Geometry check sheet. Reference: the model listing, model coordinates, mm. A direction names the side the tool comes from. Coordinates: 2 decimals unless noted, no trailing zeros. Order: outer loops, then holes, each group sorted by start corner. A loop starts at its lowest first (then second) coordinate and runs counter-clockwise, first axis right, second up. Notation, with made-up numbers: (88, -31) -> (111, -31) arc R6 ccw to (111, -26) -> close; hole circle Ø10 at (-9, -18). An arc over 180 degrees is marked (long way). Answer as CSV lines item,"result". Start each with the question number.
from build123d import *

# Parameters (mm, degrees)
SKETCH_W             = 125
SKETCH_H             = 185
PAD_DEPTH            = 5
SKETCH001_W          = 10
SKETCH001_H          = 5
PAD001_DEPTH         = 5
SKETCH002_W          = 10
SKETCH002_H          = 5
PAD002_DEPTH         = 5
SKETCH003_W          = 5
SKETCH003_H          = 10
PAD003_DEPTH         = 5
SKETCH004_R          = 15
POCKET_DEPTH         = 5.001
SKETCH005_R          = 2.5
POCKET001_DEPTH      = 0.001
POCKET001_DEPTH_BACK = 5.001
SKETCH006_R          = 2.5
POCKET002_DEPTH      = 0.001
POCKET002_DEPTH_BACK = 5.001


with BuildPart() as part:
    # Sketch → Pad (new body)
    with BuildSketch(Plane.YZ):
        with Locations((62.5, 92.5)):
            Rectangle(SKETCH_W, SKETCH_H)
    extrude(amount=PAD_DEPTH)

    # Sketch001 (on Face6 of Pad) → Pad001 (join)
    with BuildSketch(Plane.YZ.offset(5)):
        with Locations((110, 187.5)):
            Rectangle(SKETCH001_W, SKETCH001_H)
        with Locations((90, 187.5)):
            Rectangle(SKETCH001_W, SKETCH001_H)
    extrude(amount=-PAD001_DEPTH)

    # Sketch002 (on Face14 of Pad001) → Pad002 (join)
    with BuildSketch(Plane.YZ.offset(5)):
        with Locations((10, -2.5)):
            Rectangle(SKETCH002_W, SKETCH002_H)
        with Locations((30, -2.5)):
            Rectangle(SKETCH002_W, SKETCH002_H)
        with Locations((50, -2.5)):
            Rectangle(SKETCH002_W, SKETCH002_H)
        with Locations((70, -2.5)):
            Rectangle(SKETCH002_W, SKETCH002_H)
        with Locations((90, -2.5)):
            Rectangle(SKETCH002_W, SKETCH002_H)
        with Locations((110, -2.5)):
            Rectangle(SKETCH002_W, SKETCH002_H)
    extrude(amount=-PAD002_DEPTH)

    # Sketch003 (on Face38 of Pad002) → Pad003 (join)
    with BuildSketch(Plane.YZ.offset(5)):
        with Locations((-2.5, 180)):
            Rectangle(SKETCH003_W, SKETCH003_H)
        with Locations((-2.5, 160)):
            Rectangle(SKETCH003_W, SKETCH003_H)
        with Locations((-2.5, 140)):
            Rectangle(SKETCH003_W, SKETCH003_H)
        with Locations((-2.5, 120)):
            Rectangle(SKETCH003_W, SKETCH003_H)
        with Locations((-2.5, 100)):
            Rectangle(SKETCH003_W, SKETCH003_H)
    extrude(amount=-PAD003_DEPTH)

    # Sketch004 (on Face55 of Pad003) → Pocket (cut, through all)
    with BuildSketch(Plane.YZ.offset(5)):
        with Locations((30, 110)):
            Circle(SKETCH004_R)
    extrude(amount=-POCKET_DEPTH, mode=Mode.SUBTRACT)

    # Sketch005 → Pocket001 (cut, two sides)
    with BuildSketch(Plane.YZ) as pocket001_sk:
        with Locations((15, 65)):
            Circle(SKETCH005_R)
        with Locations((110, 65)):
            Circle(SKETCH005_R)
    extrude(amount=-POCKET001_DEPTH, mode=Mode.SUBTRACT)
    extrude(pocket001_sk.sketch, amount=POCKET001_DEPTH_BACK, mode=Mode.SUBTRACT)

    # Sketch006 → Pocket002 (cut, two sides)
    with BuildSketch(Plane.YZ) as pocket002_sk:
        with Locations((55, 115)):
            Circle(SKETCH006_R)
        with Locations((115, 115)):
            Circle(SKETCH006_R)
    extrude(amount=-POCKET002_DEPTH, mode=Mode.SUBTRACT)
    extrude(pocket002_sk.sketch, amount=POCKET002_DEPTH_BACK, mode=Mode.SUBTRACT)


solid = part.part
Q1. Go/stop test with flat-tipped pins: pin 1 Ø2.5 at (x, y) = (2.5, 39) entering from -Z; pin 2 Ø1.5 at (x, z) = (2.5, -3.5) entering from +Y; pin 3 Ø1.5 at (x, z) = (1.5, 108.5) entering from -Y. Record where each tip stops, or that it passes through.
Q2. Sectioned sample at D-D, the plane x = 0.95. Give the number of separate pieces and of enclosed holes in the cut face, then the cut area to 3 significant figures.
Q3. Sectioned sample at C-C, the plane y = 110. Record the cut outline in (x, z).
Q4. Access from +Z, -Z, +X, -X, +Y, -Y to the whole of each face (thin tool, end or side, straight path). Record for faces 4 (the flat face through (3, 95, 187)), 5 (the flat face through (2, 0, 110)), 6 (the flat face through (2, 20, 0)).
Q5. Sectioned sample at A-A, the plane z = 65. Record the cut outline in (x, y), then the cut area to 3 significant figures.
Q6. Thickness scan on L1, parallel to Y at x = 2.6, z = 65; L2, parallel to Z at x = 3.5, y = 110; L3, parallel to Z at x = 3, y = 30. Record the ranges inside material, lowest first.
Q7. Release check for a two-part mould opening along Z. For faces 1 (the flat face through (3, 110, -5)), 2 (the flat face through (3, 105, 187)), 3 (the cylindrical face through (2.535, 26.748, 95.357)) record: released by +Z, released by -Z, zero draft, split by the parting line, or undercut.
Q8. Sectioned sample at B-B, the plane y = 30. Record the cut outline in (x, z), then the cut area to 3 significant figures.
Geometry results:
1,pin 1,"stops at z = 0"
1,pin 2,"stops at y = 115"
1,pin 3,"stops at y = 0"
2,separate pieces,"1"
2,enclosed holes,"5"
2,area,"23,000 mm^2"
3,outline,"(0, -5) -> (5, -5) -> (5, 62.5) -> (0, 62.5) -> close; (0, 67.5) -> (5, 67.5) -> (5, 190) -> (0, 190) -> close"
4,face 4,"+Z, +X, -X"
4,face 5,"+X, -X, -Y"
4,face 6,"-Z, +X, -X"
5,outline,"(0, 0) -> (5, 0) -> (5, 12.5) -> (0, 12.5) -> close; (0, 17.5) -> (5, 17.5) -> (5, 107.5) -> (0, 107.5) -> close; (0, 112.5) -> (5, 112.5) -> (5, 125) -> (0, 125) -> close"
5,area,"575 mm^2"
6,L1,"y = 0 to 12.5, 17.5 to 107.5, 112.5 to 125"
6,L2,"z = -5 to 62.5, 67.5 to 190"
6,L3,"z = -5 to 95, 125 to 185"
7,face 1,"released by -Z"
7,face 2,"zero draft"
7,face 3,"undercut"
8,outline,"(0, -5) -> (5, -5) -> (5, 95) -> (0, 95) -> close; (0, 125) -> (5, 125) -> (5, 185) -> (0, 185) -> close"
8,area,"800 mm^2"
